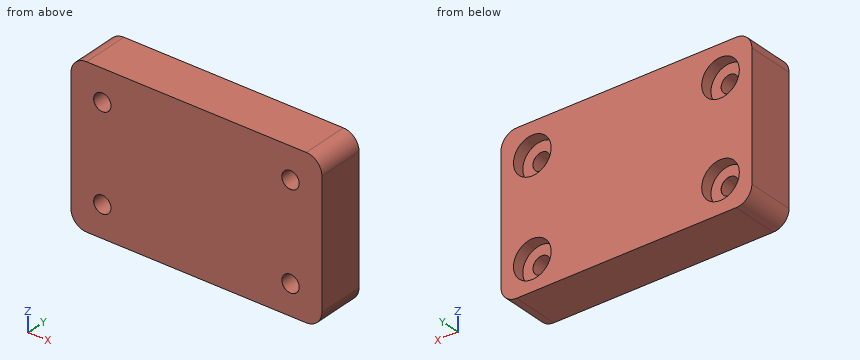
from build123d import *

# Parameters (mm, degrees)
SALIENTE_EXTRUIR1_DEPTH                     = 30
REFRENTADO_PARA_TORNILLO_CON_CABEZA_2_COUNT = 2
REFRENTADO_PARA_TORNILLO_CON_CABEZA_2_PITCH = 120.002783684
REFRENTADO_PARA_TORNILLO_CON_CABEZA_3_COUNT = 2
REFRENTADO_PARA_TORNILLO_CON_CABEZA_3_PITCH = 60
REFRENTADO_PARA_TORNILLO_CON_CABEZA_4_COUNT = 2
REFRENTADO_PARA_TORNILLO_CON_CABEZA_4_PITCH = 134.16407865


with BuildPart() as part:
    # Croquis1 → Saliente-Extruir1 (new body)
    with BuildSketch(Plane(origin=(0, 0, 0), x_dir=(1, 0, 0), z_dir=(0, 1, 0))):
        with BuildLine():
            Line((-70, -50), (70, -50))
            ThreePointArc((70, -50), (77.071067812, -47.071067812), (80, -40))
            Line((80, -40), (80, 40))
            ThreePointArc((80, 40), (77.071067812, 47.071067812), (70, 50))
            Line((70, 50), (-70, 50))
            ThreePointArc((-70, 50), (-77.071067812, 47.071067812), (-80, 40))
            Line((-80, 40), (-80, -40))
            ThreePointArc((-80, -40), (-77.071067812, -47.071067812), (-70, -50))
        make_face()
    extrude(amount=SALIENTE_EXTRUIR1_DEPTH)

    # Croquis5 → Refrentado para tornillo con cabeza troncocónica de M101 (revolve, cut)
    with BuildSketch(Plane(origin=(-60, 30, -30), x_dir=(0, 0, 1), z_dir=(1, 0, 0))):
        Polygon((0, 0), (0, 30), (5.525, 30), (5.5, 29.975), (5.5, 7.525), (5.525, 7.5), (12, 7.5), (12, 0), align=None)
    refrentado_para_tornillo_con_cabeza_tron = revolve(axis=Axis((-60, 36.35, -30), (0, -1, 0)), mode=Mode.SUBTRACT)

    # Refrentado para tornillo con cabeza  2: Refrentado para tornillo con cabeza troncocónica de M101 ×2
    with Locations(*[Vector(0.9999768031686442, 0, -0.006811249857308006) * (i * REFRENTADO_PARA_TORNILLO_CON_CABEZA_2_PITCH) for i in range(1, REFRENTADO_PARA_TORNILLO_CON_CABEZA_2_COUNT)]):
        add(refrentado_para_tornillo_con_cabeza_tron, mode=Mode.SUBTRACT)

    # Refrentado para tornillo con cabeza  3: Refrentado para tornillo con cabeza troncocónica de M101 ×2
    with Locations(*[(0, 0, i * REFRENTADO_PARA_TORNILLO_CON_CABEZA_3_PITCH) for i in range(1, REFRENTADO_PARA_TORNILLO_CON_CABEZA_3_COUNT)]):
        add(refrentado_para_tornillo_con_cabeza_tron, mode=Mode.SUBTRACT)

    # Refrentado para tornillo con cabeza  4: Refrentado para tornillo con cabeza troncocónica de M101 ×2
    with Locations(*[Vector(0.894427190999916, 0, 0.447213595499958) * (i * REFRENTADO_PARA_TORNILLO_CON_CABEZA_4_PITCH) for i in range(1, REFRENTADO_PARA_TORNILLO_CON_CABEZA_4_COUNT)]):
        add(refrentado_para_tornillo_con_cabeza_tron, mode=Mode.SUBTRACT)


solid = part.part
Could you check a few things on this model? Use its own coordinates, in mm. Give positions to 0.01 mm unless a question says otherwise; leave off trailing zeros. Write each loop counter-clockwise with the first axis right and the second up, starting at its lowest first coordinate (ties: lowest second). Pieces come first, ordered by that corner, then holes. Notation, with made-up numbers: (-13.5, 75) -> (-2.5, 75) arc R22 ccw to (-2.5, 110) -> close; hole circle Ø10 at (-39.5, 5). An arc over 180 degrees is marked (long way). Answer as a JSON object with one key per item and string values.
Q1. Suppose I cut it at D-D on y = 18. Write out the boundary of the cut face in (x, z).
Taken from the geometry:
{"outline": "(-80, -40) arc R10 ccw to (-70, -50) -> (70, -50) arc R10 ccw to (80, -40) -> (80, 40) arc R10 ccw to (70, 50) -> (-70, 50) arc R10 ccw to (-80, 40) -> close; hole circle Ø11 at (-60, -30); hole circle Ø11 at (-60, 30); hole circle Ø11 at (60, -30.82); hole circle Ø11 at (60, 30)"}
Q2. Suppose I cut it at C-C on z = -30. Count the separate pieces of the cut face and the enclosed holes in it, then the cut area to 3 significant figures.
Taken from the geometry:
{"separate pieces": "3", "enclosed holes": "0", "area": "3,950 mm²"}
Q3. Please list where these lines run through material, in increasing order: L1, parallel to Z at x = -60, y = 27.75; L2, parallel to Z at x = -60, y = 12; L3, parallel to X at y = 26.5, z = -30.
Taken from the geometry:
{"L1": "z = -50 to -42, -18 to 18, 42 to 50", "L2": "z = -50 to -35.5, -24.5 to 24.5, 35.5 to 50", "L3": "x = -80 to -72, -48 to 48.03, 71.97 to 80"}
Q4. Suppose I cut it at A-A on y = 27.75. Write out the boundary of the cut face in (x, z), then the cut area to 3 significant figures.
Taken from the geometry:
{"outline": "(-80, -40) arc R10 ccw to (-70, -50) -> (70, -50) arc R10 ccw to (80, -40) -> (80, 40) arc R10 ccw to (70, 50) -> (-70, 50) arc R10 ccw to (-80, 40) -> close; hole circle Ø24 at (-60, -30); hole circle Ø24 at (-60, 30); hole circle Ø24 at (60, -30.82); hole circle Ø24 at (60, 30)", "area": "14,100 mm²"}
Q5. Will these pins go through, and if not, where does the flat tip stop? pin 1 Ø12 at (x, z) = (-59.5, 26.5) entering from +Y; pin 2 Ø10 at (x, z) = (60, -30.82) entering from +Y.
Taken from the geometry:
{"pin 1": "stops at y = 22.5", "pin 2": "passes through"}
Q6. Suppose I cut it at B-B on x = -60. Write out the boundary of the cut face in (y, z) (3 decimals).
Taken from the geometry:
{"outline": "(0, -50) -> (30, -50) -> (30, -42) -> (22.5, -42) -> (22.5, -35.525) -> (22.475, -35.5) -> (0.025, -35.5) -> (0, -35.525) -> close; (0, -24.475) -> (0.025, -24.5) -> (22.475, -24.5) -> (22.5, -24.475) -> (22.5, -18) -> (30, -18) -> (30, 18) -> (22.5, 18) -> (22.5, 24.475) -> (22.475, 24.5) -> (0.025, 24.5) -> (0, 24.475) -> close; (0, 35.525) -> (0.025, 35.5) -> (22.475, 35.5) -> (22.5, 35.525) -> (22.5, 42) -> (30, 42) -> (30, 50) -> (0, 50) -> close"}
